Input: part model. Units: mm. Frame: model coordinates. A direction names the side the tool comes from. Coordinates: 2 decimals unless noted, no trailing zeros. Write each loop counter-clockwise with the first axis right and the second up, starting at its lowest first coordinate (ties: lowest second). Pieces come first, ordered by that corner, then holes.
1) Section query A-A (y = -10). Output: boundary loops of the cut face in (x, z).
2) Section query D-D (z = -19.5). Output: boundary loops of the cut face in (x, y), then the cut area to 3 significant figures.
3) Set-up query: faces 4 (the flat face through (4.437, 2.692, -32.3)), 5 (the flat face through (5.5, -12, -21)). Return all of +Z, -Z, +X, -X, +Y, -Y with unobstructed straight access to the full face (end or side cutting, diameter ignored); none if empty.
4) Section query C-C (x = 3.25). State how many separate pieces and enclosed holes the cut face has, then the cut area to 3 significant figures.
5) Section query B-B (z = -26.5). Output: boundary loops of the cut face in (x, y).
6) Draft query along Z for faces 1 (the cylindrical face through (4.56, -22.02, -38.8)), 2 (the flat face through (4, -10, 0)), 3 (the cylindrical face through (4.44, -15.71, -2.83)). Return one class per face: pulls with the +Z half, pulls with the -Z half, needs draft (parallel to the pull), parting line crosses it, or undercut.
7) Line query: L1, parallel to Y at x = 3.8, z = -22.5; L2, parallel to Y at x = 2.75, z = -22; L3, parallel to Z at x = 1, y = -32.5. Output: solid intervals per line, ascending.
8) Pin query (flat end, axial travel): pin 1 Ø4 at (x, y) = (4.5, -30) entering from +Z; pin 2 Ø18 at (y, z) = (-12, -20) entering from -X; pin 3 Ø1 at (x, z) = (1.5, -23.5) entering from -Y; pin 4 Ø4 at (x, y) = (4.5, -21.5) entering from -Z. Return the tip coordinate at first contact, or that it passes through.
from build123d import *

# Parameters (mm, degrees)
SKETCH1_R           = 1.3
BOSS_EXTRUDE1_DEPTH = 9
CUT_REVOLVE3_ANGLE  = 180
SKETCH8_R           = 8.1
CUT_EXTRUDE4_DEPTH  = 5.5
SKETCH9_R           = 2.25
CUT_EXTRUDE5_DEPTH  = 52.660312042
BOSS_EXTRUDE7_DEPTH = 9
CUT_REVOLVE4_ANGLE  = 180
FILLET1_R           = 6
FILLET2_R           = 4
FILLET3_R           = 3
FILLET4_R           = 3


with BuildPart() as part:
    # Sketch1 → Boss-Extrude1 (new body)
    with BuildSketch(Plane(origin=(0, 0, 0), x_dir=(0, 0, -1), z_dir=(1, 0, 0))):
        Polygon((0, -20), (22.5, -24.769696007), (45, -20), (45, 0), (22.5, 4.769696007), (0, 0), align=None)
        with Locations((22.5, -20.680807118)):
            Circle(SKETCH1_R, mode=Mode.SUBTRACT)
        with Locations((22.5, 0.680807118)):
            Circle(SKETCH1_R, mode=Mode.SUBTRACT)
        with Locations((42, -17)):
            Circle(SKETCH1_R, mode=Mode.SUBTRACT)
        with Locations((3, -17)):
            Circle(SKETCH1_R, mode=Mode.SUBTRACT)
        with Locations((3, -3)):
            Circle(SKETCH1_R, mode=Mode.SUBTRACT)
        with Locations((42, -3)):
            Circle(SKETCH1_R, mode=Mode.SUBTRACT)
    extrude(amount=BOSS_EXTRUDE1_DEPTH)

    # Sketch7 → Cut-Revolve3 (revolve, cut)
    with BuildSketch(Plane.ZY):
        with BuildLine():
            Line((-41.7, -10), (-31.3, -10))
            ThreePointArc((-31.3, -10), (-36.5, -4.8), (-41.7, -10))
        make_face()
        with BuildLine():
            Line((-13.7, -10), (-3.3, -10))
            ThreePointArc((-3.3, -10), (-8.5, -4.8), (-13.7, -10))
        make_face()
    revolve(axis=Axis((0, -10, -41.7), (0, 0, -1)), revolution_arc=CUT_REVOLVE3_ANGLE, mode=Mode.SUBTRACT)

    # Sketch8 → Cut-Extrude4 (cut)
    with BuildSketch(Plane.ZY):
        with Locations((-22.5, -10)):
            Circle(SKETCH8_R)
    extrude(amount=-CUT_EXTRUDE4_DEPTH, mode=Mode.SUBTRACT)

    # Sketch9 → Cut-Extrude5 (cut, through all)
    with BuildSketch(Plane.ZY.offset(-5.5)):
        with Locations((-22.5, -10)):
            Circle(SKETCH9_R)
    extrude(amount=-CUT_EXTRUDE5_DEPTH, mode=Mode.SUBTRACT)

    # Sketch16 → Boss-Extrude7 (add)
    with BuildSketch(Plane(origin=(9, 0, 0), x_dir=(0, 0, -1), z_dir=(1, 0, 0))):
        Polygon((38.152173913, -21.451646611), (38.152173913, -38.451646611), (23.152173913, -38.451646611), (23.152173913, -24.631443949), align=None)
    extrude(amount=-BOSS_EXTRUDE7_DEPTH)

    # Sketch17 → Cut-Revolve4 (revolve, cut)
    with BuildSketch(Plane.ZY):
        with BuildLine():
            Line((-25.452173913, -30.451646611), (-35.852173913, -30.451646611))
            ThreePointArc((-35.852173913, -30.451646611), (-30.652173913, -25.251646611), (-25.452173913, -30.451646611))
        make_face()
    revolve(axis=Axis((0, -30.451646611, -25.452173913), (0, 0, -1)), revolution_arc=CUT_REVOLVE4_ANGLE, mode=Mode.SUBTRACT)

    # Fillet1
    fillet1_edges = [part.edges().sort_by_distance(p)[0] for p in [
        (4.5, -38.451646611, -38.152173913),
        (4.5, -38.451646611, -23.152173913),
    ]]
    fillet(fillet1_edges, radius=FILLET1_R)

    # Fillet2
    fillet2_edges = [part.edges().sort_by_distance(p)[0] for p in [
        (4.5, -20, -45),
        (4.5, -20, 0),
        (4.5, 0, 0),
        (4.5, 0, -45),
    ]]
    fillet(fillet2_edges, radius=FILLET2_R)

    # Fillet3
    # the kernel refuses this fillet: 3 mm, written as the material it adds along each edge
    with BuildSketch(Plane(origin=(9, -24.631443949, -23.152173913), x_dir=(0, -0.20737808726534282, 0.9782608695650501), z_dir=(-1, 0, 0))) as fillet3_piece_1:
        with BuildLine():
            CenterArc((3.350740319, -1.340055458), FILLET3_R, 153.468795145, 38.499950409)
            Line((0.41595771, -1.96218972), (0.357262058, -1.974632405))
            Line((0.357262058, -1.974632405), (-0.058695652, -0.012442685))
            Line((-0.058695652, -0.012442685), (0, 0.06))
            ThreePointArc((0, 0.06), (0.333333333, 0.06), (0.612985194, 0.026801109))
            Line((0.612985194, 0.026801109), (0.666666667, 0))
        make_face()
    extrude(amount=9)
    with BuildSketch(Plane(origin=(9, -21.451646611, -38.152173913), x_dir=(0, -1, 0), z_dir=(-1, 0, 0))) as fillet3_piece_2:
        with BuildLine():
            CenterArc((FILLET3_R * 0.810235733018, -FILLET3_R), FILLET3_R, 90, 78.031254445)
            Line((-FILLET3_R * 0.168025136547, -FILLET3_R * 0.792621912735), (-FILLET3_R * 0.187590353938, -FILLET3_R * 0.78847435099))
            Line((-FILLET3_R * 0.187590353938, -FILLET3_R * 0.78847435099), (-FILLET3_R * 0.0162047146604, FILLET3_R * 0.02))
            Line((-FILLET3_R * 0.0162047146604, FILLET3_R * 0.02), (FILLET3_R * 0.810235733018, FILLET3_R * 0.02))
            Line((FILLET3_R * 0.810235733018, FILLET3_R * 0.02), (FILLET3_R * 0.810235733018, 0))
        make_face()
    extrude(amount=9)

    # Fillet4
    fillet4_edges = [part.edges().sort_by_distance(p)[0] for p in [
        (4.5, -24.769696007, -22.5),
    ]]
    fillet(fillet4_edges, radius=FILLET4_R)


solid = part.part
Answer:
1. outline: (0, -45) - (9, -45) - (9, -24.75) - (5.5, -24.75) - (5.5, -30.6) - (0, -30.6) - (0, -31.3) arc R5.2 cw to (0, -41.7) - close; (0, -14.4) - (5.5, -14.4) - (5.5, -20.25) - (9, -20.25) - (9, 0) - (0, 0) - (0, -3.3) arc R5.2 cw to (0, -13.7) - close
2. outline: (0, -24.13) - (9, -24.13) - (9, 4.13) - (0, 4.13) - (0, -2.48) - (5.5, -2.48) - (5.5, -17.52) - (0, -17.52) - close
2. area: 172 mm2
3. face 4: -Z, +X, -X, +Y
3. face 5: -X
4. separate pieces: 1
4. enclosed holes: 10
4. area: 931 mm2
5. outline: (0, -37.83) - (9, -37.83) - (9, 3.92) - (0, 3.92) - (0, -2.96) - (5.5, -2.96) - (5.5, -17.04) - (0, -17.04) - (0, -27.32) arc R3.13 cw to (0, -33.58) - close
6. face 1: pulls with the -Z half
6. face 2: pulls with the +Z half
6. face 3: undercut
7. L1: y = -25.47 to -21.98, -19.38 to -18.1, -1.9 to -0.62, 1.98 to 4.77
7. L2: y = -24.98 to -21.88, -19.48 to -18.08, -1.92 to -0.52, 1.88 to 4.66
7. L3: z = -38.15 to -35.33, -25.98 to -23.15
8. pin 1: stops at z = -23.15
8. pin 2: stops at x = 0
8. pin 3: stops at y = -35.53
8. pin 4: stops at z = -43.91
